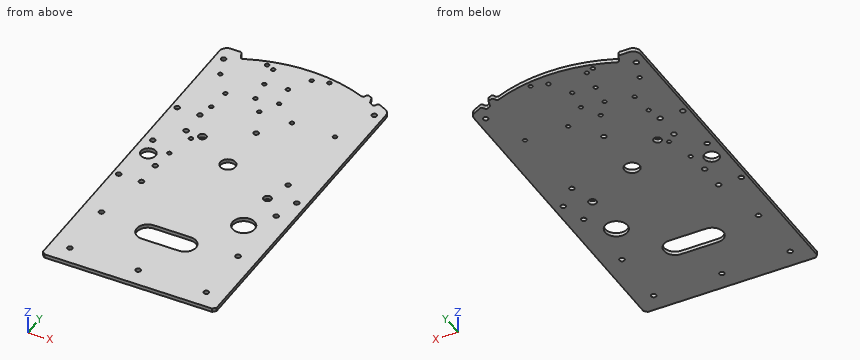
from build123d import *

# Parameters (mm, degrees)
BOSS_EXTRUDE1_DEPTH             = 3.175
SKETCH2_R                       = 6.50875
CUT_EXTRUDE1_DEPTH              = 268.458155353
F_4_CLEARANCE_HOLE1_D           = 3.4544
F_6_CLEARANCE_HOLE2_D           = 4.3053
F_4_CLEARANCE_HOLE2_D           = 3.4544
F_1_4_CLEARANCE_HOLE2_D         = 6.7564
SKETCH15_W                      = 148.719955274
SKETCH15_H                      = 114.3
BOSS_EXTRUDE2_DEPTH             = 3.175
F_6_CLEARANCE_HOLE3_D           = 4.3053
CHAMFER1_SIZE                   = 2.54
F_6_CLEARANCE_HOLE4_D           = 4.3053
F_4_CLEARANCE_HOLE3_D           = 3.4544
F_6_CLEARANCE_HOLE1_D           = 4.3053
DELETEFACE1_START               = -3.175
DELETEFACE1_OUTLINE_R           = 2.15265
DELETEFACE1_DEPTH               = 3.175
F_1_2_0_5_DIAMETER_HOLE1_D      = 12.7
F_1_4_CLEARANCE_HOLE1_D         = 6.7564
F_3_4_0_75_DIAMETER_HOLE1_D     = 19.05
F_3_4_START                     = -3.175
F_3_4_0_75_DIAMETER_SLOT1_DEPTH = 3.175
FILLET1_R                       = 1.5875
FILLET2_R                       = 6.35


# Read off the part's stored shape, not the designer's step: DeleteFace1, 3/4 (0.75) Diameter Slot1
with BuildPart() as part:
    # Sketch1 → Boss-Extrude1 (new body)
    with BuildSketch(Plane.XY):
        with BuildLine():
            Line((-37.014245685, -65.193042462), (-37.014245685, -242.993042462))
            Line((-37.014245685, -242.993042462), (111.705709589, -242.993042462))
            Line((111.705709589, -242.993042462), (111.705709589, -78.837199032))
            Line((111.705709589, -78.837199032), (100.315919098, -73.219132409))
            Line((100.315919098, -73.219132409), (98.04889923, -77.407452736))
            ThreePointArc((98.04889923, -77.407452736), (95.944511883, -76.292837527), (93.820355363, -75.216374688))
            Line((93.820355363, -75.216374688), (91.991959695, -69.073183497))
            Line((91.991959695, -69.073183497), (87.625459733, -67.171845985))
            Line((87.625459733, -67.171845985), (85.800454124, -71.570795948))
            ThreePointArc((85.800454124, -71.570795948), (33.712742218, -61.505341345), (-18.130011823, -72.76464689))
            Line((-18.130011823, -72.76464689), (-20.055584156, -68.408779876))
            Line((-20.055584156, -68.408779876), (-21.49685031, -65.148469374))
            Line((-21.49685031, -65.148469374), (-28.430836618, -65.168386968))
            Line((-28.430836618, -65.168386968), (-37.014245685, -65.193042462))
        make_face()
    extrude(amount=-BOSS_EXTRUDE1_DEPTH)

    # Sketch2 → Cut-Extrude1 (cut, through all)
    with BuildSketch(Plane.XY):
        with Locations((35.268404938, -193.371995598)):
            Circle(SKETCH2_R)
    extrude(amount=-CUT_EXTRUDE1_DEPTH, mode=Mode.SUBTRACT)

    # #4 Clearance Hole1 (through all)
    with Locations(Plane.XY):
        with Locations((41.939844363, -71.488811907), (9.789450293, -73.011273216), (90.488583573, -124.967078721), (53.658735514, -125.072870965), (25.338848707, -124.341705755), (-9.634401538, -135.888162669), (55.145248163, -67.700310852), (3.101953943, -70.270684884)):
            Hole(F_4_CLEARANCE_HOLE1_D / 2)

    # #6 Clearance Hole2 (through all)
    with Locations(Plane.XY):
        with Locations((-29.394245685, -79.071995598), (104.085709589, -87.326995598), (35.695953558, -148.921995598), (26.485754315, -79.071995598)):
            Hole(F_6_CLEARANCE_HOLE2_D / 2)

    # #4 Clearance Hole2 (through all)
    with Locations(Plane.XY):
        with Locations((-8.073739309, -116.319383279), (-22.812224861, -96.782058908), (-10.478566815, -201.738004366), (-4.603970045, -177.980497914)):
            Hole(F_4_CLEARANCE_HOLE2_D / 2)

    # 1/4 Clearance Hole2 (through all)
    with Locations(Plane.XY):
        with Locations((81.551198953, -216.670082089)):
            Hole(F_1_4_CLEARANCE_HOLE2_D / 2)

    # Sketch15 → Boss-Extrude2 (add, through all)
    with BuildSketch(Plane.XY):
        with Locations((37.345731952, -300.143042462)):
            Rectangle(SKETCH15_W, SKETCH15_H)
    extrude(amount=-BOSS_EXTRUDE2_DEPTH)

    # #6 Clearance Hole3 (through all)
    with Locations(Plane.XY):
        with Locations((-29.076745685, -193.371995598), (103.768209589, -211.243042462), (87.470455138, -194.579117263), (97.722907594, -232.841790729)):
            Hole(F_6_CLEARANCE_HOLE3_D / 2)

    # Chamfer1
    chamfer1_edges = [part.edges().sort_by_distance(p)[0] for p in [
        (-37.014245685, -357.293042462, -1.5875),
        (111.705709589, -357.293042462, -1.5875),
    ]]
    chamfer(chamfer1_edges, length=CHAMFER1_SIZE)

    # #6 Clearance Hole4 (through all)
    with Locations(Plane.XY):
        with Locations((95.830709589, -341.418042462), (37.345731952, -341.418042462), (-21.139245685, -341.418042462), (95.830709589, -290.618042462), (-21.139245685, -290.618042462)):
            Hole(F_6_CLEARANCE_HOLE4_D / 2)

    # #4 Clearance Hole3 (through all)
    with Locations(Plane.XY):
        with Locations((31.354393952, -89.701374676), (12.464345577, -92.164821934), (14.927792835, -111.054870309), (33.81784121, -108.591423051)):
            Hole(F_4_CLEARANCE_HOLE3_D / 2)

    # #6 Clearance Hole1 (through all)
    with Locations(Plane.XY):
        with Locations((-12.436474575, -171.172679278), (-12.436474575, -148.947679278), (-31.934245685, -148.947679278), (-31.934245685, -242.800679278), (-12.436474575, -242.800679278), (-12.436474575, -220.575679278)):
            Hole(F_6_CLEARANCE_HOLE1_D / 2)

    # DeleteFace1 outline → DeleteFace1 (add)
    with BuildSketch(Plane.XY.offset(DELETEFACE1_START)):
        with Locations((26.485754315, -79.071995598)):
            Circle(DELETEFACE1_OUTLINE_R)
    extrude(amount=DELETEFACE1_DEPTH)

    # 1/2 (0.5) Diameter Hole1 (through all)
    with Locations(Plane.XY):
        with Locations((-24.314245685, -209.463179278)):
            Hole(F_1_2_0_5_DIAMETER_HOLE1_D / 2)

    # 1/4 Clearance Hole1 (through all)
    with Locations(Plane.XY):
        with Locations((1.896126146, -171.892035997)):
            Hole(F_1_4_CLEARANCE_HOLE1_D / 2)

    # 3/4 (0.75) Diameter Hole1 (through all)
    with Locations(Plane.XY):
        with Locations((81.551198953, -254.770082089)):
            Hole(F_3_4_0_75_DIAMETER_HOLE1_D / 2)

    # 3/4 (0.75) Diameter Slot1 outline → 3/4 (0.75) Diameter Slot1 (cut)
    with BuildSketch(Plane.XY.offset(F_3_4_START)):
        with BuildLine():
            Line((21.470731952, -305.605683453), (53.220731952, -305.605683453))
            ThreePointArc((53.220731952, -305.605683453), (62.745731952, -296.080683453), (53.220731952, -286.555683453))
            Line((53.220731952, -286.555683453), (21.470731952, -286.555683453))
            ThreePointArc((21.470731952, -286.555683453), (11.945731952, -296.080683453), (21.470731952, -305.605683453))
        make_face()
    extrude(amount=F_3_4_0_75_DIAMETER_SLOT1_DEPTH, mode=Mode.SUBTRACT)

    # Fillet1
    fillet1_edges = [part.edges().sort_by_distance(p)[0] for p in [
        (-21.49685031, -65.148469374, -1.5875),
        (-18.130011823, -72.76464689, -1.5875),
        (85.800454124, -71.570795948, -1.5875),
        (87.625459733, -67.171845985, -1.5875),
        (91.991959695, -69.073183497, -1.5875),
        (93.820355363, -75.216374688, -1.5875),
        (98.04889923, -77.407452736, -1.5875),
        (100.315919098, -73.219132409, -1.5875),
    ]]
    fillet(fillet1_edges, radius=FILLET1_R)

    # Fillet2
    fillet2_edges = [part.edges().sort_by_distance(p)[0] for p in [
        (111.705709589, -78.837199032, -1.5875),
        (-37.014245685, -65.193042462, -1.5875),
    ]]
    fillet(fillet2_edges, radius=FILLET2_R)


solid = part.part
Verification items for the finished model (mm, model axes). Coordinates: 2 decimals unless noted, no trailing zeros. One line per question, with ' | ' between items.
1) Material ranges on L1, parallel to X at y = -292.5, z = -1.45; L2, parallel to Y at x = 105.5, z = -1.4; L3, parallel to Y at x = 4, z = -2.85, recorded low to high.
Solutions:
L1: -37.01 to -22.18, -20.09 to 12.64, 62.05 to 94.79, 96.88 to 111.71 | L2: -357.29 to -212.52, -209.96 to -88.95, -85.7 to -75.78 | L3: -357.29 to -174.54, -169.25 to -71.75, -68.8 to -65.24
2) Sectioned sample at A-A on z = -1.5. State how many separate pieces and enclosed holes the cut face has, then the cut area to 3 significant figures.
Solutions:
separate pieces: 1 | enclosed holes: 40 | area: 41,300 mm^2
3) Depth check by flat-ended pin: pin 1 Ø5 at (x, y) = (-29.39, -79.07) entering from -Z (3 decimals). Enter the tip coordinate at first touch or a pass-through.
Solutions:
pin 1: z = -3.175
